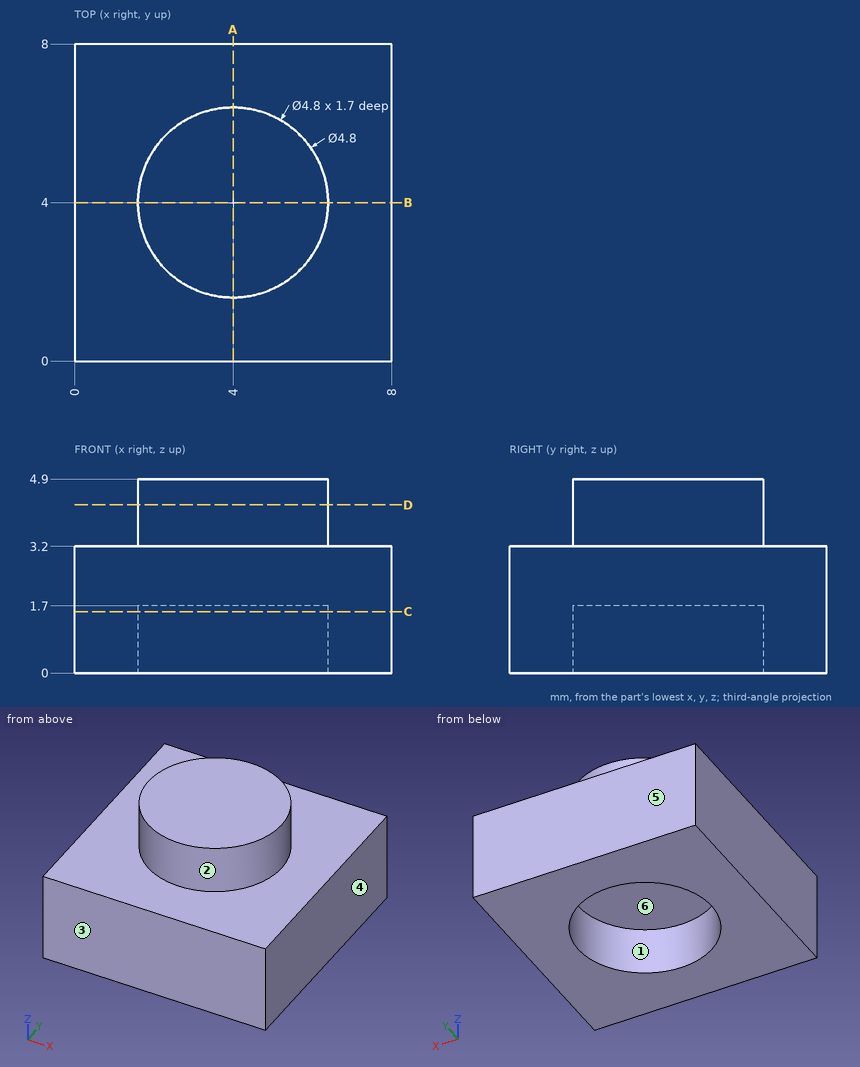
Here's the drawing with two shaded views (mm, measured from the low corner). I have some questions. A direction names the side the tool comes from. Round coordinates to 2 decimals unless told otherwise and drop trailing zeros. Write each loop counter-clockwise with the first axis right and the second up, starting at its lowest first coordinate (ties: lowest second). Pieces come first, ordered by that corner, then holes. Notation, with made-up numbers: M 64,14.25 L 73,14.25 A14 ccw 73,26.25 Z; hole C -35,83.5 d11. An arc over 180 degrees is marked long. Answer in a Markdown table with one row per item. Add a question column.
Q1. On a 3-axis mill with a long thin cutter (end or side, diameter ignored), from which of +Z, -Z, +X, -X, +Y, -Y can I reach the whole of each face in a straight line? I mean the marked faces 1, 2 and 3. Say none if no direction works.
Q2. Imagine slicing it at C-C (z = 1.55). Please give me the cut outline in (x, y), then the cut area to 3 significant figures.
Q3. If I drill on line 1 (Y direction, x = 4, z = 0.4); line 2 (Z direction, x = 1.5, y = 5.5); line 3 (X direction, y = 3.5, z = 1.25), over which ranges is the centre line in solid material (lowest first)? Write a range as from..to.
Q4. If we mould it in two halves opening along Y, with no side actions, what happens to the marked faces 4, 5 and 6? For each: +Y half, -Y half, draft (parallel to the pull), parting line (faces both ways), or undercut.
Q5. Imagine slicing it at D-D (z = 4.25). Please give me the cut outline in (x, y).
Q6. Will this pin go through, and if not, where does the flat tip stop? pin 1 Ø1 at (x, y) = (1, 4) entering from +Z.
Q7. Imagine slicing it at A-A (x = 4). Please give me the cut outline in (y, z).
Values:
| question | item | result |
|---|---|---|
| 1 | face 1 | -Z |
| 1 | face 2 | +Z |
| 1 | face 3 | +Z, -Z, +X, -X, -Y |
| 2 | outline | M 0,0 L 8,0 L 8,8 L 0,8 Z; hole C 4,4 d4.8 |
| 2 | area | 45.9 mm^2 |
| 3 | line 1 | 0..1.6, 6.4..8 |
| 3 | line 2 | 0..3.2 |
| 3 | line 3 | 0..1.65, 6.35..8 |
| 4 | face 4 | draft |
| 4 | face 5 | +Y half |
| 4 | face 6 | undercut |
| 5 | outline | C 4,4 d4.8 |
| 6 | pin 1 | z = 3.2 |
| 7 | outline | M 0,0 L 1.6,0 L 1.6,1.7 L 6.4,1.7 L 6.4,0 L 8,0 L 8,3.2 L 6.4,3.2 L 6.4,4.9 L 1.6,4.9 L 1.6,3.2 L 0,3.2 Z |
